Here's how the part is built. I have some questions about the finished solid (model axes, mm). A direction names the side the tool comes from. Round coordinates to 2 decimals unless told otherwise and drop trailing zeros. Write each loop counter-clockwise with the first axis right and the second up, starting at its lowest first coordinate (ties: lowest second). Pieces come first, ordered by that corner, then holes. Notation, with made-up numbers: (51.5, 23) - (96.5, 23) arc R17 cw to (96.5, 36) - close; hole circle Ø7 at (12, 37). An arc over 180 degrees is marked (long way). One line per item, written item: value. Start each with the question number.
Item 1: Imagine slicing it at D-D, the plane z = 1.65. Please give me the cut outline in (x, y), then the cut area to 3 significant figures.
Item 2: For faces 1 (the face through (0, -1, 1.08)), 2 (the face through (-1.954, -6.837, 0.086)), which set-ups out of +Z, -Z, +X, -X, +Y, -Y let a thin tool reach every point of the face, with its end or its side?
Item 3: Imagine slicing it at A-A, the plane x = 0. Please give me the cut outline in (y, z) (1 decimal).
Item 4: If I drill on line 1 (X direction, y = 0, z = 1.75); line 2 (X direction, y = 0, z = -1.5); line 3 (Y direction, x = 0, z = 1.65), over which ranges is the centre line in solid material (lowest first)?
Item 5: Imagine slicing it at C-C, the plane y = -13. Please give me the cut outline in (x, z).
Item 6: Thinking about a two-plate mould opening in Y: for faces 3 (the face through (-0.096, -0.434, 1.513)), 4 (the face through (0, -3.175, 0)), 5 (the face through (0, -1, -1.08)), which applies, released by +Y, released by -Y, zero draft, split by the parting line, or undercut?
Item 7: Imagine slicing it at B-B, the plane z = 0. Please give me the cut outline in (x, y) (3 decimals), then the cut area to 3 significant figures.
```python
from build123d import *

# Parameters (mm, degrees)
CUT_EXTRUDE1_DEPTH      = 17.064109466
CUT_EXTRUDE1_DEPTH_BACK = 17.064109466
SKETCH2_W               = 2.159
SKETCH2_H               = 5.314367205
CUT_EXTRUDE2_DEPTH      = 17.064109466
CUT_EXTRUDE2_DEPTH_BACK = 17.064109466
SKETCH3_R               = 0.4445


with BuildPart() as part:
    # Sketch1 one side → Revolve1 (revolve)
    with BuildSketch(Plane.XY):
        with BuildLine():
            Line((1.9558, -13.8684), (1.9558, 0))
            ThreePointArc((1.9558, 0), (1.382959443, 1.382959443), (0, 1.9558))
            Line((0, 1.9558), (0, -15.8242))
            ThreePointArc((0, -15.8242), (1.382959443, -15.251359443), (1.9558, -13.8684))
        make_face()
    revolve(axis=Axis((0, 0, 0), (0, -1, 0)))

    # Sketch2 → Cut-Extrude1 (cut, two sides: drawn at the far end of the back side and taken through both)
    with BuildSketch(Plane(origin=(0, 0, 0), x_dir=(0, 0, -1), z_dir=(1, 0, 0)).offset(-CUT_EXTRUDE1_DEPTH_BACK)):
        with Locations((0, -0.517816398)):
            Rectangle(SKETCH2_W, SKETCH2_H)
    extrude(amount=CUT_EXTRUDE1_DEPTH + CUT_EXTRUDE1_DEPTH_BACK, mode=Mode.SUBTRACT)

    # Sketch3 → Cut-Extrude2 (cut, two sides: drawn at the far end of the back side and taken through both)
    with BuildSketch(Plane.XY.offset(-CUT_EXTRUDE2_DEPTH_BACK)):
        Circle(SKETCH3_R)
    extrude(amount=CUT_EXTRUDE2_DEPTH + CUT_EXTRUDE2_DEPTH_BACK, mode=Mode.SUBTRACT)


solid = part.part
```
Values follow:
1. outline: (-1.05, -13.87) arc R1.05 ccw to (1.05, -13.87) - (1.05, 0) arc R1.05 ccw to (-1.05, 0) - close; hole circle Ø0.89 at (0, 0)
1. area: 32.0 mm^2
2. face 1: +X, -X, +Y
2. face 2: +Y, -Y
3. outline: (-13.9, -2) - (-0.4, -2) - (-0.4, -1.1) - (-3.2, -1.1) - (-3.2, 1.1) - (-0.4, 1.1) - (-0.4, 2) - (-13.9, 2) arc R2 ccw to start; (0.4, -1.9) arc R2 ccw to (1.6, -1.1) - (0.4, -1.1) - close; (0.4, 1.1) - (1.6, 1.1) arc R2 ccw to (0.4, 1.9) - close
4. line 1: x = -0.87 to -0.44, 0.44 to 0.87
4. line 2: x = -1.26 to -0.44, 0.44 to 1.26
4. line 3: y = -14.92 to -0.44, 0.44 to 1.05
5. outline: circle Ø3.91 at (0, 0)
6. face 3: undercut
6. face 4: released by +Y
6. face 5: zero draft
7. outline: (-1.956, -13.868) arc R1.956 ccw to (1.956, -13.868) - (1.956, -3.175) - (-1.956, -3.175) - close
7. area: 47.8 mm^2
